Work out the finished part from the listing and answer in its coordinate system (mm). Face numbers are marked on the shaded views. Round coordinates to 2 decimals unless told otherwise and drop trailing zeros. Loops run counter-clockwise (first coordinate to the right, second up) from the corner with the lowest first, then second, coordinate; pieces in that order, holes last. Notation, with made-up numbers: (30.5, 18) - (49.5, 18) arc R26 cw to (49.5, 57) - close; hole circle Ø3 at (-13, -35.75). An arc over 180 degrees is marked (long way). Answer as CSV lines item,"result". Start each with the question number.
Q1. Each of these flat-tipped pins is pushed along its axis until it touches: pin 1 Ø2 at (x, z) = (-15, 3) entering from +Y; pin 2 Ø2 at (y, z) = (16.5, 2) entering from -X; pin 3 Ø1 at (x, z) = (8, 2.5) entering from -Y. Where does it stop, or does it pass through?
Q2. The mould has two halves that part along Y. Classify the marked faces 1, 2 and 3: +Y half, -Y half, draft (parallel to the pull), parting line (faces both ways), or undercut.
Q3. Section B-B on z = 4.35 is taken. Write down the section's boundary in (x, y).
Q4. Section D-D on x = -6 is taken. Write down the section's boundary in (y, z).
Q5. Section C-C on y = -15.5 is taken. Write down the section's boundary in (x, z).
Q6. Section A-A on x = 0 is taken. Write down the section's boundary in (y, z).
Q7. Straight lines are drawn through the part: L1, parallel to X at y = 5.5, z = 2.4; L2, parallel to X at y = 4, z = 3.1; L3, parallel to Y at x = -10, z = 3.6. For each, find the intervals that lie inside material, in ascending order. Write a range as [from, to].
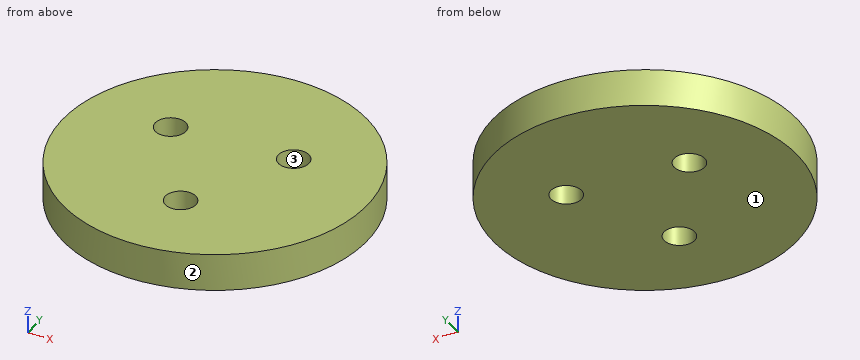
Autodesk Inventor part; units mm, degrees
ref_plane "YZ Plane" through (0, 0, 0) normal (1, 0, 0) x (0, 1, 0)
ref_plane "XZ Plane" through (0, 0, 0) normal (0, 1, 0) x (-1, 0, 0)
ref_plane "XY Plane" through (0, 0, 0) normal (0, 0, 1) x (1, 0, 0)
sketch "Sketch1" plane through (0, 0, 0) normal (0, 0, 1) x (1, 0, 0)
  circle A0 centre (-0.671, 10.228) radius 3.5
  circle A1 centre (-8.5222, -5.6951) radius 3.5
  circle A2 centre (9.1932, -4.5329) radius 3.5
  circle A3 centre (0, 0) radius 15
  circle A4 centre (8.5222, 5.6951) radius 2
  circle A5 centre (0.671, -10.228) radius 2
  circle A6 centre (-9.1932, 4.5329) radius 2
  circle A7 centre (20.0905, -24.1532) radius 3.75
  circle A8 centre (-30.4505, 7.7314) radius 3.75
  circle A9 centre (-2.0567, 31.3493) radius 3.75
  circle A10 centre (-16.7628, -26.571) radius 3.75
  circle A11 centre (29.1794, 11.6435) radius 3.75
  circle A12 centre (0, 0) radius 23.3333
  arc A13 (-39.4862, -1.0454) -> (-35.737, -7.6127) centre (-31.489, -0.8337) ccw
  arc A14 (-34.2512, -12.7254) -> (-35.737, -7.6127) centre (-37.861, -11.0021) ccw
  arc A15 (-34.2512, -12.7254) -> (-33.8969, -20.2792) centre (-27.0317, -16.172) ccw
  arc A16 (-33.8969, -20.2792) -> (36.2558, -15.6768) centre (0, 0) ccw
  arc A17 (36.2558, -15.6768) -> (35.6202, -8.1415) centre (28.9129, -12.5018) ccw
  arc A18 (36.4252, -2.8784) -> (35.6202, -8.1415) centre (38.9739, -5.9614) ccw
  arc A19 (36.4252, -2.8784) -> (39.2843, 4.1223) centre (31.328, 3.2874) ccw
  arc A20 (39.2843, 4.1223) -> (-39.4862, -1.0454) centre (0, 0) ccw
  line L0 (0, 23.3333) -> (0, 22.3333)
  circle A21 centre (0, 0) radius 22.3333
  point P0 (0, 0)
  dimension "d0" = 1
extrude "Extrusion1" add sketch "Sketch1" along normal blind 3.5 contours A0 | A1 | A2 | A3 | A21
sketch "Sketch2" plane through (0, 0, 0) normal (0, 0, -1) x (-1, 0, 0)
  circle A0 centre (0, 0) radius 22.3333
  circle A1 centre (-8.5222, 5.6951) radius 2
  circle A2 centre (-0.671, -10.228) radius 2
  circle A3 centre (9.1932, 4.5329) radius 2
  circle A4 centre (-8.5222, 5.6951) radius 2.25
  circle A5 centre (9.1932, 4.5329) radius 2.25
  circle A6 centre (-0.671, -10.228) radius 2
  circle A7 centre (-0.671, -10.228) radius 2.25
  point P0 (0, 0)
  dimension "d3" = 4.5
  dimension "d4" = 4.5
  dimension "d5" = 4.5
extrude "Extrusion2" cut sketch "Sketch2" against normal through all contours A1 | A2 | A3 | A4 | A5 | A7
sketch "Szkic3" plane through (0, 0, 3.5) normal (0, 0, 1) x (1, 0, 0)
  circle A0 centre (0.671, -10.228) radius 2.25
  circle A1 centre (-9.1932, 4.5329) radius 2.25
  circle A2 centre (8.5222, 5.6951) radius 2.25
  circle A3 centre (0, 0) radius 22.3333
  point P0 (0, 0)
extrude "Wyciągnięcie proste3" add sketch "Szkic3" along normal blind 2
properties part number "kółko"
Findings:
1,pin 1,"stops at y = 17.4"
1,pin 2,"stops at x = -16.08"
1,pin 3,"stops at y = -21.04"
2,face 1,"draft"
2,face 2,"parting line"
2,face 3,"undercut"
3,outline,"circle Ø44.67 at (0, 0); hole circle Ø4.5 at (-9.19, 4.53); hole circle Ø4.5 at (0.67, -10.23); hole circle Ø4.5 at (8.52, 5.7)"
4,outline,"(-21.51, 0) - (21.51, 0) - (21.51, 5.5) - (-21.51, 5.5) - close"
5,outline,"(-16.08, 0) - (16.08, 0) - (16.08, 5.5) - (-16.08, 5.5) - close"
6,outline,"(-22.33, 0) - (-12.38, 0) - (-12.38, 5.5) - (-22.33, 5.5) - close; (-8.08, 0) - (22.33, 0) - (22.33, 5.5) - (-8.08, 5.5) - close"
7,L1,"x = [-21.65, -11.22], [-7.16, 6.28], [10.76, 21.65]"
7,L2,"x = [-21.97, -11.38], [-7.01, 7.04], [10, 21.97]"
7,L3,"y = [-19.97, 2.43], [6.63, 19.97]"
